Check sheet for the modelled part. Datum: model origin and axes. Units: mm. Face numbers are marked on the shaded views. A direction names the side the tool comes from. Give positions to 0.01 mm unless a question says otherwise; leave off trailing zeros. Write each loop counter-clockwise with the first axis right and the second up, starting at its lowest first coordinate (ties: lowest second). Pieces come first, ordered by that corner, then holes. Notation, with made-up numbers: (32, -21) -> (75, -21) arc R27 cw to (75, 6) -> close; hole circle Ø10 at (87.25, 69.25). An arc over 180 degrees is marked (long way). Use a Markdown table: item, result. Add a question column.
1. Gauge pin test, flat ends, axial feed: P1, Ø8, axis at x = -8.5, y = 45, coming from the -Z side; P2, Ø12, axis at y = 48, z = -11, coming from the -X side; P3, Ø10, axis at y = 39.5, z = -26, coming from the +X side. Record the tip position at first contact, or that the pin passes through.
2. Set-up check for the marked faces 1, 2, 3 and 4: record each of +Z, -Z, +X, -X, +Y, -Y from which the full face is reachable in a straight line by a thin tool's end or side.
3. Cross-section at C-C (x = 0). Enter the section's corners in (y, z) (3 decimals), then the cut area to 3 significant figures.
4. Cross-section at B-B (y = 0). Enter the section's corners in (x, z) (3 decimals), then the cut area to 3 significant figures.
5. Cross-section at A-A (z = -19). Enter the section's corners in (x, y) (3 decimals).
6. Cross-section at D-D (x = -19.5). Enter the section's corners in (y, z), then the cut area to 3 significant figures.
7. Scan lines: probe 1 along Y at (x, z) = (0, -16) (3 decimals); probe 2 along Y at (x, z) = (0, -44) (3 decimals); probe 3 along X at (y, z) = (4, -38.5). Record each from-to range of solid material in increasing order. Write a range as [from, to].
from build123d import *

# Parameters (mm, degrees)
SKETCH1_W           = 124
SKETCH1_H           = 48
SKETCH1_R           = 4.525
BOSS_EXTRUDE1_DEPTH = 55.25
SKETCH2_W           = 70
SKETCH2_H           = 33
BOSS_EXTRUDE2_DEPTH = 33
CHAMFER1_SIZE       = 15
CHAMFER1_SIZE2      = 25.980762114


with BuildPart() as part:
    # Sketch1 → Boss-Extrude1 (new body)
    with BuildSketch(Plane.XY):
        Rectangle(SKETCH1_W, SKETCH1_H)
        Circle(SKETCH1_R, mode=Mode.SUBTRACT)
    extrude(amount=-BOSS_EXTRUDE1_DEPTH)

    # Sketch2 → Boss-Extrude2 (add)
    with BuildSketch(Plane(origin=(0, 24, 0), x_dir=(1, 0, 0), z_dir=(0, 1, 0))):
        with Locations((-26.99, 26.5)):
            Rectangle(SKETCH2_W, SKETCH2_H)
    extrude(amount=BOSS_EXTRUDE2_DEPTH)

    # Chamfer1
    chamfer1_edges = [part.edges().sort_by_distance(p)[0] for p in [
        (62, 0, -55.25),
    ]]
    chamfer1_side = [part.faces().sort_by_distance(p)[0] for p in [
        (0, 22.670338389, -55.25),
    ]]
    chamfer(chamfer1_edges, length=CHAMFER1_SIZE, length2=CHAMFER1_SIZE2, reference=chamfer1_side[0])


solid = part.part
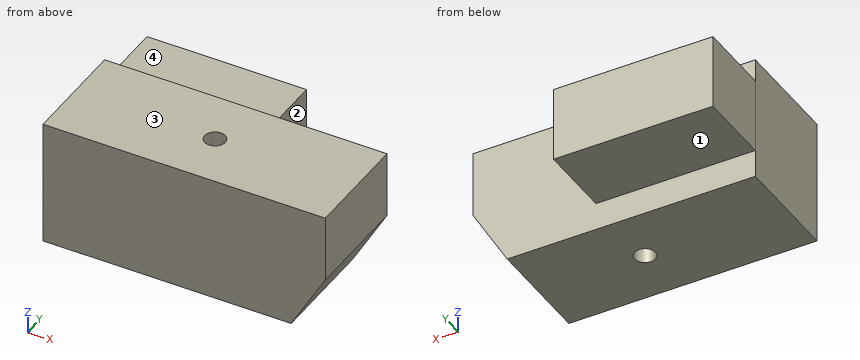
Worked answers:
| question | item | result |
|---|---|---|
| 1 | P1 | stops at z = -43 |
| 1 | P2 | stops at x = -61.99 |
| 1 | P3 | stops at x = 8.01 |
| 2 | face 1 | -Z, +X, -X, +Y |
| 2 | face 2 | +Z, -Z, +X, +Y |
| 2 | face 3 | +Z, +X, -X, +Y, -Y |
| 2 | face 4 | +Z, +X, -X, +Y |
| 3 | outline | (-24, -55.25) -> (-4.525, -55.25) -> (-4.525, 0) -> (-24, 0) -> close; (4.525, -55.25) -> (24, -55.25) -> (24, -43) -> (57, -43) -> (57, -10) -> (24, -10) -> (24, 0) -> (4.525, 0) -> close |
| 3 | area | 3,240 mm² |
| 4 | outline | (-62, -55.25) -> (-4.525, -55.25) -> (-4.525, 0) -> (-62, 0) -> close; (4.525, -55.25) -> (47, -55.25) -> (62, -29.269) -> (62, 0) -> (4.525, 0) -> close |
| 4 | area | 6,160 mm² |
| 5 | outline | (-62, -24) -> (62, -24) -> (62, 24) -> (8.01, 24) -> (8.01, 57) -> (-61.99, 57) -> (-61.99, 24) -> (-62, 24) -> close; hole circle Ø9.05 at (0, 0) |
| 6 | outline | (-24, -55.25) -> (24, -55.25) -> (24, -43) -> (57, -43) -> (57, -10) -> (24, -10) -> (24, 0) -> (-24, 0) -> close |
| 6 | area | 3,740 mm² |
| 7 | probe 1 | y = [-24, -4.525], [4.525, 57] |
| 7 | probe 2 | y = [-24, -4.525], [4.525, 24] |
| 7 | probe 3 | x = [-62, -2.12], [2.12, 56.67] |
